from build123d import *

# Parameters (mm, degrees)
EXTRUDE1_DEPTH     = 18.25625
FILLET1_R          = 6.35
SKETCH3_R          = 7.9375
CUT_EXTRUDE1_DEPTH = 37.5125
SKETCH4_R          = 5.55625
CUT_EXTRUDE2_DEPTH = 13.7


with BuildPart() as part:
    # Sketch1 → Extrude1 (new body, symmetric)
    with BuildSketch(Plane.XY):
        with BuildLine():
            Line((-63.5, 0), (63.5, 0))
            Line((63.5, 0), (63.5, 12.7))
            Line((63.5, 12.7), (31.75, 12.7))
            Line((31.75, 12.7), (25.4, 39.382325452))
            ThreePointArc((25.4, 39.382325452), (0, 59.446883653), (-25.4, 39.382325452))
            Line((-25.4, 39.382325452), (-31.75, 12.7))
            Line((-31.75, 12.7), (-63.5, 12.7))
            Line((-63.5, 12.7), (-63.5, 0))
        make_face()
    extrude(amount=EXTRUDE1_DEPTH, both=True)

    # Fillet1
    fillet1_edges = [part.edges().sort_by_distance(p)[0] for p in [
        (-31.75, 12.7, 0),
        (31.75, 12.7, 0),
    ]]
    fillet(fillet1_edges, radius=FILLET1_R)

    # Sketch3 → Cut-Extrude1 (cut, through all)
    with BuildSketch(Plane.XY.offset(18.25625)):
        with Locations((0, 33.3375)):
            Circle(SKETCH3_R)
    extrude(amount=-CUT_EXTRUDE1_DEPTH, mode=Mode.SUBTRACT)

    # Sketch4 → Cut-Extrude2 (cut, through all)
    with BuildSketch(Plane(origin=(0, 12.7, 0), x_dir=(-1, 0, 0), z_dir=(0, 1, 0))):
        with Locations((-47.625, 0)):
            Circle(SKETCH4_R)
        with Locations((47.625, 0)):
            Circle(SKETCH4_R)
    extrude(amount=-CUT_EXTRUDE2_DEPTH, mode=Mode.SUBTRACT)


solid = part.part
Can you work these out from the model? Positions are in its coordinate system, mm. A direction names the side the tool comes from. Coordinates: 2 decimals unless noted, no trailing zeros. Order: outer loops, then holes, each group sorted by start corner. A loop starts at its lowest first (then second) coordinate and runs counter-clockwise, first axis right, second up. Notation, with made-up numbers: (-5, 83) - (33, 83) arc R19 ccw to (33, 101) - close; hole circle Ø1 at (74, -6.5). An arc over 180 degrees is marked (long way). Answer as a JSON object with one key per item and string values. Group by question number.
Q1. We'd pull the mould along Z, two halves only. Please class faces 1 (the face through (-1, 24, 18.256)), 2 (the face through (-1, 24, -18.256)), 3 (the face through (53.176, 6.439, 0.244)), 4 (the face through (-1, 0, 0)): +Z half, -Z half, draft (parallel to the pull), parting line (faces both ways), or undercut.
Q2. I need wall thicknesses on line 1 (Y direction, x = 44, z = 8.5); line 2 (Y direction, x = 3, z = -10.5); line 3 (X direction, y = 39, z = 11). Which ranges of each line are inside material? Lowest first, please. Write a range as from..to.
Q3. Imagine slicing it at C-C (y = 8). Please give me the cut outline in (x, z) (1 decimal), and give its area (3 significant figures).
Q4. Imagine slicing it at A-A (z = 0). Give the number of separate pieces and of enclosed holes in the cut face, and give its area (3 significant figures).
Q5. On a 3-axis mill with a long thin cutter (end or side, diameter ignored), from which of +Z, -Z, +X, -X, +Y, -Y can I reach the whole of each face in a straight line? I mean faces 5 (the face through (63.5, 6, 0)), 6 (the face through (53, 12.7, 4)), 7 (the face through (-53, 12.7, 4)). Say none if no direction works.
Q6. Imagine slicing it at B-B (x = 5). Please give me the cut outline in (y, z).
Q7. Will these pins go through, and if not, where does the flat tip stop? P1, Ø3, axis at y = 38, z = -7.5, coming from the +X side; P2, Ø1.5, axis at y = 22.5, z = -11, coming from the +X side; P3, Ø2, axis at x = -5.5, z = 4, coming from the -Y side; P4, Ø3, axis at y = 36, z = -13.5, coming from the +X side.
Determined:
{
 "1": {"face 1": "+Z half", "face 2": "-Z half", "face 3": "undercut", "face 4": "draft"},
 "2": {"line 1": "y = 0..12.7", "line 2": "y = 0..25.99, 40.69..59.27", "line 3": "x = -25.49..-5.56, 5.56..25.49"},
 "3": {"outline": "(-63.5, -18.3) - (63.5, -18.3) - (63.5, 18.3) - (-63.5, 18.3) - close; hole circle Ø11.1 at (-47.6, 0); hole circle Ø11.1 at (47.6, 0)", "area": "4,440 mm2"},
 "4": {"separate pieces": "3", "enclosed holes": "1", "area": "3,430 mm2"},
 "5": {"face 5": "+Z, -Z, +X, +Y, -Y", "face 6": "+Z, -Z, +X, +Y", "face 7": "+Z, -Z, -X, +Y"},
 "6": {"outline": "(0, -18.26) - (27.17, -18.26) - (27.17, 18.26) - (0, 18.26) - close; (39.5, -18.26) - (58.96, -18.26) - (58.96, 18.26) - (39.5, 18.26) - close"},
 "7": {"P1": "stops at x = 26.09", "P2": "stops at x = 29.6", "P3": "stops at y = 0", "P4": "stops at x = 26.56"}
}
